```python
from build123d import *

# Parameters (mm, degrees)
SKETCH_1_R               = 72.5
SKETCH_1_R_2             = 60
EXTRUDE_1_DEPTH          = 3
SKETCH_2_R               = 2.5
EXTRUDE_2_DEPTH          = 6
PATTERN_CIRCULAR_1_COUNT = 5
EXTRUDE_START            = 3
SKETCH_3_R               = 60
EXTRUDE_3_DEPTH          = 3
SKETCH_4_R               = 3.5
CUT_EXTRUDE_1_DEPTH      = 10
SKETCH_5_R               = 18.027756377
CUT_EXTRUDE_2_DEPTH      = 1.5


with BuildPart() as part:
    # 草图1 → 凸台-拉伸1 (new body)
    with BuildSketch(Plane(origin=(0, 0, 0), x_dir=(1, 0, 0), z_dir=(0, 1, 0))):
        with Locations(Location((0, 0, 0), (0, 0, 270))):
            Circle(SKETCH_1_R)
        with Locations(Location((0, 0, 0), (0, 0, 270))):
            Circle(SKETCH_1_R_2, mode=Mode.SUBTRACT)
    extrude(amount=EXTRUDE_1_DEPTH)

    # 草图2 → 凸台-拉伸2 (add)
    with BuildSketch(Plane(origin=(0, 0, 0), x_dir=(1, 0, 0), z_dir=(0, 1, 0))):
        with Locations(Location((0, 66.25, 0), (0, 0, 270))):
            Circle(SKETCH_2_R)
    extrude_2 = extrude(amount=-EXTRUDE_2_DEPTH)

    # 阵列(圆周)1: 凸台-拉伸2 ×5 about axis
    pattern_circular_1_axis = Axis((0, 0, 0), (0, 1, 0))
    for i in range(1, PATTERN_CIRCULAR_1_COUNT):
        add(extrude_2.rotate(pattern_circular_1_axis, i * 360 / PATTERN_CIRCULAR_1_COUNT))

    # 草图3 → 凸台-拉伸3 (add)
    with BuildSketch(Plane.XZ.offset(6).offset(EXTRUDE_START)):
        with BuildLine():
            Line((10, 112.979589711), (10, 97.979589711))
            ThreePointArc((10, 97.979589711), (12.254033308, 91.655034391), (18, 88.18163074))
            ThreePointArc((18, 88.18163074), (0, -90), (-18, 88.18163074))
            ThreePointArc((-18, 88.18163074), (-12.254033308, 91.655034391), (-10, 97.979589711))
            Line((-10, 97.979589711), (-10, 112.979589711))
            ThreePointArc((-10, 112.979589711), (0, 122.979589711), (10, 112.979589711))
        make_face()
        with Locations(Location((0, 0, 0), (0, 0, 90))):
            Circle(SKETCH_3_R, mode=Mode.SUBTRACT)
    extrude(amount=-EXTRUDE_3_DEPTH)

    # 草图4 → 切除-拉伸1 (cut)
    with BuildSketch(Plane(origin=(0, 0, 0), x_dir=(1, 0, 0), z_dir=(0, 1, 0))):
        with Locations(Location((0, -112.979589711, 0), (0, 0, 90))):
            Circle(SKETCH_4_R)
    extrude(amount=-CUT_EXTRUDE_1_DEPTH, mode=Mode.SUBTRACT)

    # 草图5 → 切除-拉伸2 (cut)
    with BuildSketch(Plane(origin=(0, -6, 0), x_dir=(1, 0, 0), z_dir=(0, 1, 0))):
        with Locations((0, -112.979589711)):
            Circle(SKETCH_5_R)
    extrude(amount=-CUT_EXTRUDE_2_DEPTH, mode=Mode.SUBTRACT)


solid = part.part
```
Can you work these out from the model? Positions are in its coordinate system, mm. A direction names the side the tool comes from. Coordinates: 2 decimals unless noted, no trailing zeros. Order: outer loops, then holes, each group sorted by start corner. A loop starts at its lowest first (then second) coordinate and runs counter-clockwise, first axis right, second up. Notation, with made-up numbers: (-34, 86) -> (-28, 86) arc R26 cw to (-28, 124) -> close; hole circle Ø7 at (21.25, 36.5). An arc over 180 degrees is marked (long way). Write each question's results on one line, items separated by ' | '.
Item 1: I want a section at D-D, the plane z = -66.25. Write out the boundary of the cut face in (x, y), then the cut area to 3 significant figures.
Results are:
outline: (-60.92, -9) -> (60.92, -9) -> (60.92, -6) -> (2.5, -6) -> (2.5, 0) -> (29.45, 0) -> (29.45, 3) -> (-29.45, 3) -> (-29.45, 0) -> (-2.5, 0) -> (-2.5, -6) -> (-60.92, -6) -> close | area: 572 mm²
Item 2: I want a section at B-B, the plane x = 0. Write out the boundary of the cut face in (y, z).
Results are:
outline: (-9, -90) -> (-6, -90) -> (-6, -68.75) -> (0, -68.75) -> (0, -72.5) -> (3, -72.5) -> (3, -60) -> (0, -60) -> (0, -63.75) -> (-6, -63.75) -> (-6, -60) -> (-9, -60) -> close; (-9, 60) -> (-6, 60) -> (-6, 94.95) -> (-7.5, 94.95) -> (-7.5, 109.48) -> (-9, 109.48) -> close; (-9, 116.48) -> (-7.5, 116.48) -> (-7.5, 122.98) -> (-9, 122.98) -> close; (0, 60) -> (3, 60) -> (3, 72.5) -> (0, 72.5) -> close
Item 3: I'm going to push flat-ended pins straight in: pin 1 Ø16 at (x, z) = (1, 104) entering from +Y; pin 2 Ø6 at (y, z) = (1, -53.5) entering from -X; pin 3 Ø5 at (y, z) = (-1.5, -45.5) entering from +X. Where does each tip first touch, or does it pass through?
Results are:
pin 1: y = -7.5 | pin 2: x = -52.02 | pin 3: x = 58
Item 4: If we mould it in two halves opening along Y, with no side actions, what happens to faces 4 (the face through (-18.7, -6, -57.4)), 5 (the face through (-0.22, -8.26, 122.977)), 6 (the face through (0, -7.5, 109))? For each: +Y half, -Y half, draft (parallel to the pull), parting line (faces both ways), or undercut.
Results are:
face 4: undercut | face 5: draft | face 6: +Y half
Item 5: Which directions (+Z, -Z, +X, -X, +Y, -Y) give clear straight access to the entire face, cutting with the end or side of a thin tool? Please do faces 1 (the face through (1.341, -8.24, 109.746)), 2 (the face through (65.28, -2.96, -19.43)), 3 (the face through (21.78, 1.48, 69.15)).
Results are:
face 1: +Y, -Y | face 2: none | face 3: +Y
Item 6: I want a section at A-A, the plane z = 0. Write out the boundary of the cut face in (x, y).
Results are:
outline: (-90, -9) -> (-60, -9) -> (-60, -6) -> (-90, -6) -> close; (-72.5, 0) -> (-60, 0) -> (-60, 3) -> (-72.5, 3) -> close; (60, -9) -> (90, -9) -> (90, -6) -> (60, -6) -> close; (60, 0) -> (72.5, 0) -> (72.5, 3) -> (60, 3) -> close
Item 7: I want a section at C-C, the plane x = 56. Write out the boundary of the cut face in (y, z), then the cut area to 3 significant figures.
Results are:
outline: (-9, -70.46) -> (-6, -70.46) -> (-6, -21.54) -> (-9, -21.54) -> close; (-9, 21.54) -> (-6, 21.54) -> (-6, 70.46) -> (-9, 70.46) -> close; (0, -46.05) -> (3, -46.05) -> (3, -21.54) -> (0, -21.54) -> close; (0, 21.54) -> (3, 21.54) -> (3, 46.05) -> (0, 46.05) -> close | area: 441 mm²
Item 8: If I drill on line 1 along Y through (x, z) = (64, -1.5); line 2 along X through (y, z) = (1.8, 0); line 3 along Y through (x, z) = (73.5, 39), over which ranges is the centre line in solid material (lowest first)?
Results are:
line 1: -9 to -6, 0 to 3 | line 2: -72.5 to -60, 60 to 72.5 | line 3: -9 to -6
